Design review of the part built by this model. Coordinates are the model's own, in mm. Face numbers are marked on the shaded views. A direction names the side the tool comes from. Round coordinates to 2 decimals unless told otherwise and drop trailing zeros. Loops run counter-clockwise (first coordinate to the right, second up) from the corner with the lowest first, then second, coordinate; pieces in that order, holes last. Notation, with made-up numbers: (-16.75, 81) -> (22.25, 81) arc R27 cw to (22.25, 99) -> close; hole circle Ø8 at (58.5, 79.5). An arc over 180 degrees is marked (long way). Answer as CSV lines item,"result". Start each with the question number.
(1) Take a section at B-B, the plane z = -9. Write out the cut boundary in (x, y), and give its area (3 significant figures).
(2) To check wall thickness, follow line 1 (Z direction, x = -25.5, y = -6.25); line 2 (X direction, y = -5.75, z = -40); line 3 (Y direction, x = -35.5, z = -61.5). State the ranges of each line that lie inside material, in increasing order. Write a range as from..to.
(3) Machinability: for the marked faces 5 and 6, which of the approach directions +Z, -Z, +X, -X, +Y, -Y give a long, thin tool a straight path to every point of the face, cutting with its end or side? Answer none if there is none.
(4) For P1, Ø3, axis at y = -1, z = -33, coming from the -X side; P2, Ø0.8, axis at x = -35.5, y = -1.5, coming from the +Z side; P3, Ø4, axis at x = -59, z = -38.5, coming from the +Y side, all flat-tipped, find the tip position at first contact; note any pin that passes through.
(5) Draft analysis for pull direction Z (two halves, no side actions). For the marked faces 1, 2, 3 and 4, state which applies: +Z half, -Z half, draft (parallel to the pull), parting line (faces both ways), or undercut.
(6) Take a section at A-A, the plane y = -7. Write out the cut boundary in (x, z).
(7) Take a section at C-C, the plane x = -83. Write out the cut boundary in (y, z).
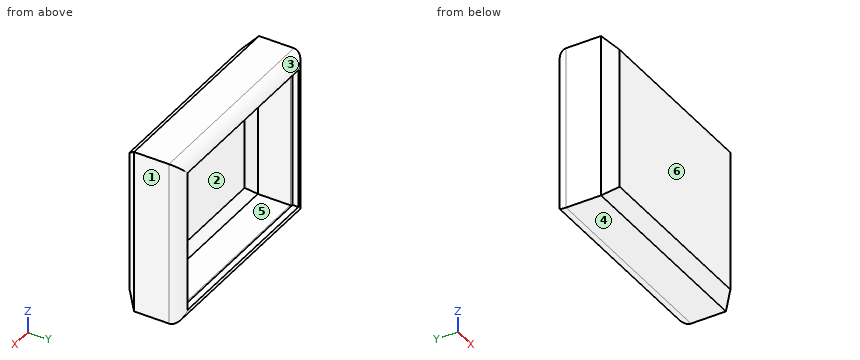
from build123d import *

# Parameters (mm, degrees)
F0_W     = 89.0572415665
F0_H     = 72.2243338823
F1_DEPTH = 25.4
F2_SIZE  = 5.08
F3_R     = 5.08
F4_T     = -2.54


# Not quite as in the source:
# - a shell that OpenCascade refuses in one call is made with other operations: the cavity is built on its own and cut out


with BuildPart() as f1:
    # F0 (on Front) → F1 (new body)
    with BuildSketch(Plane.XZ):
        with Locations((-52.9469675384, -36.1121669412)):
            Rectangle(F0_W, F0_H)
    extrude(amount=F1_DEPTH)

    # F2
    f2_edges = [f1.edges().sort_by_distance(p)[0] for p in [
        (-97.475588, -25.4, -36.112167),
        (-52.946968, -25.4, 0),
        (-8.418347, -25.4, -36.112167),
        (-52.946968, -25.4, -72.224334),
    ]]
    chamfer(f2_edges, length=F2_SIZE)

    # F3
    f3_edges = [f1.edges().sort_by_distance(p)[0] for p in [
        (-8.418347, 0, -36.112167),
        (-52.946968, 0, 0),
        (-97.475588, 0, -36.112167),
        (-52.946968, 0, -72.224334),
    ]]
    fillet(f3_edges, radius=F3_R)

    # F4: a shell. OpenCascade refuses it in one call, so the cavity is built on its own and cut out:
    # the body offset inwards by the wall thickness, plus a prism from it out through each open face.
    f4_core = offset(f1.part, amount=F4_T, mode=Mode.PRIVATE)
    f4_exits = [f4_core.faces().sort_by_distance(p)[0] for p in [
        (-52.946968, -2.54, -36.112167),
    ]]
    add(f4_core, mode=Mode.SUBTRACT)
    extrude(f4_exits, amount=-F4_T, mode=Mode.SUBTRACT)


solid = f1.part
The answers:
1,outline,"(-97.48, -20.32) -> (-92.4, -25.4) -> (-13.5, -25.4) -> (-8.42, -20.32) -> (-8.42, -5.08) arc R5.08 ccw to (-13.5, 0) -> (-13.5, -2.54) arc R2.54 cw to (-10.96, -5.08) -> (-10.96, -19.27) -> (-14.55, -22.86) -> (-91.34, -22.86) -> (-94.94, -19.27) -> (-94.94, -5.08) arc R2.54 cw to (-92.4, -2.54) -> (-92.4, 0) arc R5.08 ccw to (-97.48, -5.08) -> close"
1,area,"334 mm²"
2,line 1,"-72.22..-69.68, -2.54..0"
2,line 2,"-97.48..-94.94, -10.96..-8.42"
2,line 3,"-25.4..-22.86"
3,face 5,"none"
3,face 6,"+Z, -Z, +X, -X, -Y"
4,P1,"x = -96.77"
4,P2,"z = -1.12"
4,P3,"y = -22.86"
5,face 1,"draft"
5,face 2,"undercut"
5,face 3,"+Z half"
5,face 4,"-Z half"
6,outline,"(-97.48, -72.22) -> (-8.42, -72.22) -> (-8.42, 0) -> (-97.48, 0) -> close; hole (-94.94, -69.68) -> (-10.96, -69.68) -> (-10.96, -2.54) -> (-94.94, -2.54) -> close"
7,outline,"(-25.4, -67.14) -> (-20.32, -72.22) -> (-5.08, -72.22) arc R5.08 ccw to (0, -67.14) -> (-2.54, -67.14) arc R2.54 cw to (-5.08, -69.68) -> (-19.27, -69.68) -> (-22.86, -66.09) -> (-22.86, -6.13) -> (-19.27, -2.54) -> (-5.08, -2.54) arc R2.54 cw to (-2.54, -5.08) -> (0, -5.08) arc R5.08 ccw to (-5.08, 0) -> (-20.32, 0) -> (-25.4, -5.08) -> close"
